Input: part model. Units: mm. Frame: model coordinates. Give positions to 0.01 mm unless a question says otherwise; leave off trailing zeros. Answer in a Markdown table with one row per item. Add a question column.
1. Mould query, pull axis Y, two halves, no side actions, for faces 1 (the face through (21.671, -137.985, 40.905)), 2 (the face through (12.16, -126.63, 40.9)). Classes: released by +Y, released by -Y, zero draft, split by the parting line, or undercut.
2. Ray query, line 1 (Z direction, x = 18, y = -142.5); line 2 (Y direction, x = 10, z = 40.4); line 3 (X direction, y = -133, z = 40.7). Return the intervals inside material, ascending. Write a range as [from, to].
3. Contact query for flat-ended pins moving along their axis: pin 1 (5 mm diameter, centred on x = 31.5, y = -144.5, fed in from -Z); pin 2 (14.5 mm diameter, centred on x = 20.5, y = -142, fed in from +Z); pin 3 (1 mm diameter, centred on y = -130.5, z = 41, fed in from -X). Output: stop coordinate, or through.
```python
from build123d import *

# Parameters (mm, degrees)
SKETCH2_R           = 15
SKETCH2_R_2         = 1.5
BOSS_EXTRUDE1_DEPTH = 2
FILLET1_R           = 0.5
FILLET3_R           = 0.5


with BuildPart() as part:
    # Sketch2 → Boss-Extrude1 (new body)
    with BuildSketch(Plane(origin=(-0.007077674, -0.003066892, 41.897062416), x_dir=(0.837169553, 0.546943422, 0.00018146), z_dir=(0.00016893, 7.3201e-05, -0.999999983))):
        with Locations((-55.821998493, 127.304785363)):
            Circle(SKETCH2_R)
        with Locations((-55.821998493, 127.304785363)):
            Circle(SKETCH2_R_2, mode=Mode.SUBTRACT)
    extrude(amount=BOSS_EXTRUDE1_DEPTH)

    # Fillet1
    fillet1_edges = [part.edges().sort_by_distance(p)[0] for p in [
        (10.331416884, -145.31438544, 41.888172015),
    ]]
    fillet(fillet1_edges, radius=FILLET1_R)

    # Fillet3
    fillet3_edges = [part.edges().sort_by_distance(p)[0] for p in [
        (10.331754744, -145.314239039, 39.888172049),
    ]]
    fillet(fillet3_edges, radius=FILLET3_R)


solid = part.part
```
Answer:
| question | item | result |
|---|---|---|
| 1 | face 1 | undercut |
| 1 | face 2 | split by the parting line |
| 2 | line 1 | z = [39.89, 41.89] |
| 2 | line 2 | y = [-144.78, -129.44] |
| 2 | line 3 | x = [8.46, 37.32] |
| 3 | pin 1 | stops at z = 39.89 |
| 3 | pin 2 | stops at z = 41.89 |
| 3 | pin 3 | stops at x = 9.19 |
